Design review of the part built by this model. Coordinates are the model's own, in mm. Round coordinates to 2 decimals unless told otherwise and drop trailing zeros. Order: outer loops, then holes, each group sorted by start corner. A loop starts at its lowest first (then second) coordinate and runs counter-clockwise, first axis right, second up. Notation, with made-up numbers: M 35.5,89 L 93.5,89 A23 cw 93.5,105 Z; hole C 81.5,-24 d7. An arc over 180 degrees is marked long. Use a Markdown table: item, result. Add a question column.
(1) For pin 1 (12 mm diameter, centred on x = -6.5, z = -1, fed in from -Y); pin 2 (0.6 mm diameter, centred on x = -43, y = 1, fed in from -Z); pin 3 (1 mm diameter, centred on y = 1, z = -9, fed in from -X); pin 4 (1 mm diameter, centred on x = -43.5, y = 0.5, fed in from +Z), all flat-tipped, find the tip position at first contact; note any pin that passes through.
(2) To check wall thickness, follow probe 1 along X at (y, z) = (0.45, -6.75); probe 2 along X at (y, z) = (1.1, -1.75). State the ranges of each line that lie inside material, in increasing order. Write a range as from..to.
(3) Take a section at A-A (y = 0.35). Write out the cut boundary in (x, z).
(4) Take a section at B-B (z = -3.25). Write out the cut boundary in (x, y).
Autodesk Inventor part; units mm, degrees
ref_plane "YZ Plane" through (0, 0, 0) normal (1, 0, 0) x (0, 1, 0)
ref_plane "XZ Plane" through (0, 0, 0) normal (0, 1, 0) x (-1, 0, 0)
ref_plane "XY Plane" through (0, 0, 0) normal (0, 0, 1) x (1, 0, 0)
sketch "Sketch1" plane through (0, 0, 0) normal (0, 1, 0) x (-1, 0, 0)
  line L0 (42.5071, 12.299) -> (-23.7769, 12.299)
  line L1 (-23.7769, 12.299) -> (-23.7769, -12.701)
  line L2 (-23.7769, -12.701) -> (42.5071, -12.701)
  line L3 (42.5071, -12.701) -> (42.5071, 12.299)
  line L4 (-23.7769, 0.9818) -> (-25.7769, 0.9818)
  line L5 (-25.7769, 0.9818) -> (-25.7769, -1.0182)
  line L6 (-25.7769, -1.0182) -> (-23.7769, -1.0182)
  line L7 (-23.7769, -1.0182) -> (-23.7769, 0.9818)
  line L8 (44.5071, -1.0182) -> (42.5071, -1.0182)
  line L9 (42.5071, -1.0182) -> (42.5071, 0.9818)
  line L10 (42.5071, 0.9818) -> (44.5071, 0.9818)
  line L11 (44.5071, 0.9818) -> (44.5071, -1.0182)
  point P0 (0, 0)
  dimension "d0" = 66.284
  dimension "d1" = 25
  dimension "d2" = 2
  dimension "d3" = 2
  dimension "d11" = 2
  dimension "d12" = 2
extrude "Extrusion1" add sketch "Sketch1" along normal blind 2
sketch "Sketch2" plane through (0, 2, 0) normal (0, 1, 0) x (1, 0, 0)
  circle A0 centre (8.7493, 7.4985) radius 1
  line L0 (8.7493, 7.4985) -> (-24.4607, 7.4985)
  circle A1 centre (-24.4607, 7.4985) radius 1
  point P0 (0, 0)
  dimension "d6" = 2
  dimension "d7" = 33.21
  dimension "d8" = 2
extrude "Extrusion2" cut sketch "Sketch2" against normal blind 2
properties part number "Lclamp2"
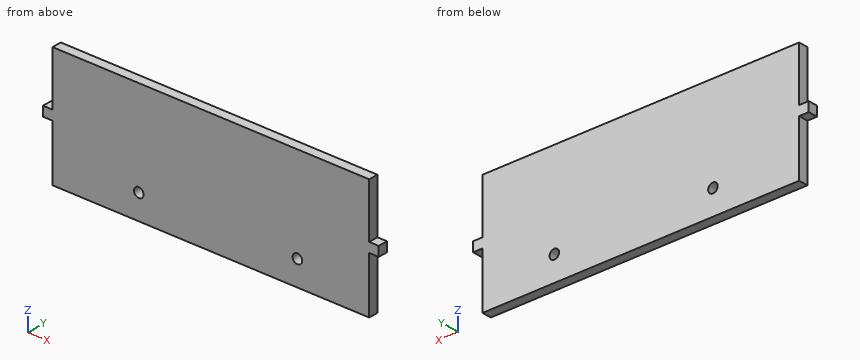
Verdict:
| question | item | result |
|---|---|---|
| 1 | pin 1 | stops at y = 0 |
| 1 | pin 2 | stops at z = -1.02 |
| 1 | pin 3 | stops at x = -42.51 |
| 1 | pin 4 | stops at z = 0.98 |
| 2 | probe 1 | x = -42.51..-25.12, -23.8..8.09, 9.41..23.78 |
| 2 | probe 2 | x = -42.51..23.78 |
| 3 | outline | M -44.51,-1.02 L -42.51,-1.02 L -42.51,-12.7 L 23.78,-12.7 L 23.78,-1.02 L 25.78,-1.02 L 25.78,0.98 L 23.78,0.98 L 23.78,12.3 L -42.51,12.3 L -42.51,0.98 L -44.51,0.98 Z; hole C -24.46,-7.5 d2; hole C 8.75,-7.5 d2 |
| 4 | outline | M -42.51,0 L 23.78,0 L 23.78,2 L -42.51,2 Z |
